```python
from build123d import *

# Parameters (mm, degrees)
F1_DEPTH  = 80
F2_R      = 12
F3_DEPTH  = 25
F5_R      = 20
F6_DEPTH  = 50
F7_R      = 6
F8_R      = 5
F9_R      = 8
F10_DEPTH = 20.001


with BuildPart() as f1:
    # F0 (on Front) → F1 (new body)
    with BuildSketch(Plane.XZ):
        Polygon((0, 65), (0, 0), (120, 0), (120, 8), (80, 8), (80, 20), (15, 20), (15, 65), align=None)
    extrude(amount=-F1_DEPTH)

    # F2 (on face) → F3 (cut)
    with BuildSketch(Plane.YZ.offset(15)):
        with BuildLine():
            Line((0, 65), (0, 20))
            Line((0, 20), (18.2297518911, 52.2904962177))
            ThreePointArc((18.2297518911, 52.2904962177), (27.3956833871, 61.5900718554), (40, 65))
            Line((40, 65), (0, 65))
        make_face()
        with BuildLine():
            Line((61.7702481089, 52.2904962177), (80, 20))
            Line((80, 20), (80, 65))
            Line((80, 65), (40, 65))
            ThreePointArc((40, 65), (52.6043166129, 61.5900718554), (61.7702481089, 52.2904962177))
        make_face()
        with Locations((40, 40)):
            Circle(F2_R)
    extrude(amount=-F3_DEPTH, mode=Mode.SUBTRACT)

    # F5 (on face) → F6 (cut, symmetric)
    with BuildSketch(Plane(origin=(0, 0, 0), x_dir=(0, 1, 0), z_dir=(0.7660444431, 0, -0.6427876097))):
        with Locations((41.4580069482, 0)):
            Circle(F5_R)
    extrude(amount=F6_DEPTH, both=True, mode=Mode.SUBTRACT)

    # F7
    f7_edges = [f1.edges().sort_by_distance(p)[0] for p in [
        (80, 40, 8),
    ]]
    fillet(f7_edges, radius=F7_R)

    # F8
    f8_edges = [f1.edges().sort_by_distance(p)[0] for p in [
        (60, 0, 0),
        (60, 80, 0),
    ]]
    fillet(f8_edges, radius=F8_R)

    # F9 (on face) → F10 (cut, through all)
    with BuildSketch(Plane.XY.offset(20)):
        with Locations((65.5771933797, 57)):
            Circle(F9_R)
        with Locations((65.5771933797, 23)):
            Circle(F9_R)
    extrude(amount=-F10_DEPTH, mode=Mode.SUBTRACT)


solid = f1.part
```
Source: CAD feature listing. Evaluate the final solid. Frame: model axes, mm. A direction names the side the tool comes from. Give positions to 0.01 mm unless a question says otherwise; leave off trailing zeros. Write each loop counter-clockwise with the first axis right and the second up, starting at its lowest first coordinate (ties: lowest second). Pieces come first, ordered by that corner, then holes.
1. Material intervals for line 1 along Z through (x, y) = (94.5, 11.5); line 2 along X through (y, z) = (70.5, 17.5); line 3 along X through (y, z) = (22.5, 53.5), sorted ascending.
2. Section query B-B (x = 77.5). Return the cut outline in (y, z), then the cut area to 3 significant figures.
3. Section query A-A (y = 38). Return the cut outline in (x, z), then the cut area to 3 significant figures.
4. Section query D-D (y = 23). Return the cut outline in (x, z), then the cut area to 3 significant figures.
5. Pull-direction query (Z, two-part tool) for faces 1 (the face through (59, 40, 0)), 2 (the face through (81.711, 40.56, 9.804)), 3 (the face through (7.605, 51.085, 35.404)), 4 (the face through (0, 31, 26)); classes: +Z half, -Z half, draft (parallel to the pull), parting line (faces both ways), or undercut.
6. First-contact query: pin 1 (18.5 mm diameter, centred on x = 65.58, y = 23, fed in from +Z); pin 2 (9.5 mm diameter, centred on x = 65.58, y = 57, fed in from +Z); pin 3 (4 mm diameter, centred on y = 32.5, z = 18, fed in from -X); pin 4 (8 mm diameter, centred on x = 12.5, z = 25, fed in from +Y). Flat tips, straight axial feed; report the tip coordinate or a pass-through.
7. Access query for faces 5 (the face through (48, 39, 20)), 6 (the face through (64.536, 64.932, 10.14)). Directions: +Z, -Z, +X, -X, +Y, -Y. A direction counts if a zero-diameter tool reaches every point of the face in a straight line with its end or side. Return the directions, or none.
8. Section query C-C (z = 40). Return the cut outline in (x, y), then the cut area to 3 significant figures.
Output values:
1. line 1: z = 0 to 8
1. line 2: x = 0 to 80
1. line 3: x = 0 to 15
2. outline: (0, 5) arc R5 ccw to (5, 0) - (75, 0) arc R5 ccw to (80, 5) - (80, 20) - (0, 20) - close
2. area: 1,590 mm2
3. outline: (0, 25.71) - (30.65, 0) - (120, 0) - (120, 8) - (86, 8) arc R6 cw to (80, 14) - (80, 20) - (15, 20) - (15, 28.17) - (0, 28.17) - close; (0, 51.83) - (15, 51.83) - (15, 64.92) - (0, 64.92) - close
3. area: 1,850 mm2
4. outline: (0, 10.05) - (11.98, 0) - (57.58, 0) - (57.58, 20) - (15, 20) - (15, 58.33) - (0, 58.33) - close; (73.58, 0) - (120, 0) - (120, 8) - (86, 8) arc R6 cw to (80, 14) - (80, 20) - (73.58, 20) - close
4. area: 2,120 mm2
5. face 1: -Z half
5. face 2: +Z half
5. face 3: undercut
5. face 4: draft
6. pin 1: stops at z = 20
6. pin 2: passes through
6. pin 3: stops at x = 3.44
6. pin 4: stops at y = 79.44
7. face 5: +Z, +X, +Y, -Y
7. face 6: +Z, -Z
8. outline: (0, 11.29) - (15, 11.29) - (15, 28) - (0, 28) - close; (0, 52) - (15, 52) - (15, 68.71) - (0, 68.71) - close
8. area: 501 mm2
